Input: part model. Units: mm. Frame: model coordinates. Round coordinates to 2 decimals unless told otherwise and drop trailing zeros. Loops run counter-clockwise (first coordinate to the right, second up) from the corner with the lowest first, then second, coordinate; pieces in that order, holes last. Notation, with made-up numbers: (-10.5, 60) - (16.5, 60) arc R23 ccw to (16.5, 79) - close; hole circle Ø4 at (36.5, 39.5). An arc over 180 degrees is marked (long way). Write each question's results on one line, items separated by ' | '.
from build123d import *

# Parameters (mm, degrees)
SKETCH008_R      = 5
EXTRUDE002_DEPTH = 10


with BuildPart() as extrude002:
    # Sketch008 (on Face5 of Cut002) → Extrude002 (new body)
    with BuildSketch(Plane.XY.offset(1)):
        with Locations((35, 0)):
            Circle(SKETCH008_R)
        with Locations((0, 35)):
            Circle(SKETCH008_R)
        with Locations((-35, 0)):
            Circle(SKETCH008_R)
        with Locations((0, -35)):
            Circle(SKETCH008_R)
        with Locations((0, 55)):
            Circle(SKETCH008_R)
        with Locations((55, 0)):
            Circle(SKETCH008_R)
        with Locations((0, -55)):
            Circle(SKETCH008_R)
        with Locations((-55, 0)):
            Circle(SKETCH008_R)
        with Locations((-24.748737, 24.748737)):
            Circle(SKETCH008_R)
        with Locations((-24.748737, -24.748737)):
            Circle(SKETCH008_R)
        with Locations((24.748737, -24.748737)):
            Circle(SKETCH008_R)
        with Locations((24.748737, 24.748737)):
            Circle(SKETCH008_R)
        with Locations((-47.631397, 27.5)):
            Circle(SKETCH008_R)
        with Locations((-27.5, 47.631397)):
            Circle(SKETCH008_R)
        with Locations((27.5, 47.631397)):
            Circle(SKETCH008_R)
        with Locations((47.631397, 27.5)):
            Circle(SKETCH008_R)
        with Locations((47.631397, -27.5)):
            Circle(SKETCH008_R)
        with Locations((27.5, -47.631397)):
            Circle(SKETCH008_R)
        with Locations((-27.5, -47.631397)):
            Circle(SKETCH008_R)
        with Locations((-47.631397, -27.5)):
            Circle(SKETCH008_R)
    extrude(amount=-EXTRUDE002_DEPTH)


with BuildPart() as cone003:
    # Cone003 → Cone003 (revolve)
    with BuildSketch(Plane(origin=(0, 0, 1), x_dir=(1, 0, 0), z_dir=(0, -1, 0))):
        Polygon((0, 0), (69, 0), (70, 9), (0, 9), align=None)
    revolve(axis=Axis((0, 0, 1), (0, 0, 1)))


with BuildPart() as simple_bottom:
    # Cone002 → Cone002 (revolve)
    with BuildSketch(Plane.XZ):
        Polygon((0, 0), (70, 0), (71, 10), (0, 10), align=None)
    revolve(axis=Axis((0, 0, 0), (0, 0, 1)))

    # Cut002: cut Cone003
    add(cone003.part, mode=Mode.SUBTRACT)

    # Cut003: cut Extrude002
    add(extrude002.part, mode=Mode.SUBTRACT)


solid = simple_bottom.part
1. Section query A-A, the plane x = 0. Output: boundary loops of the cut face in (y, z), plus the area to 3 significant figures.
Answer:
outline: (-71, 10) - (-70, 0) - (-60, 0) - (-60, 1) - (-69, 1) - (-70, 10) - close; (-50, 0) - (-40, 0) - (-40, 1) - (-50, 1) - close; (-30, 0) - (30, 0) - (30, 1) - (-30, 1) - close; (40, 0) - (50, 0) - (50, 1) - (40, 1) - close; (60, 0) - (70, 0) - (71, 10) - (70, 10) - (69, 1) - (60, 1) - close | area: 119 mm^2
2. Line query: line 1 (X direction, y = -51, z = 0.5); line 2 (Y direction, x = 27.5, z = 0.6); line 3 (X direction, y = -49, z = 5). Output: solid intervals per line, ascending. Write a range as [from, to].
Answer:
line 1: [-48.02, -31.19], [-23.81, -3], [3, 23.81], [31.19, 48.02] | line 2: [-64.44, -52.63], [-42.63, -28.92], [-20.57, 20.57], [28.92, 42.63], [52.63, 64.44] | line 3: [-50.69, -49.21], [49.21, 50.69]
3. Contact query for flat-ended pins moving along their axis: pin 1 (2 mm diameter, centred on x = -43.5, z = 4.5, fed in from +Y); pin 2 (1.5 mm diameter, centred on x = -37, z = 6, fed in from +Y); pin 3 (5 mm diameter, centred on x = -4.5, y = 2.5, fed in from +Z). Output: stop coordinate, or through.
Answer:
pin 1: y = 56.2 | pin 2: y = 60.59 | pin 3: z = 1
4. Mould query, pull axis X, two halves, no side actions, for faces 1 (the conical face through (-69.995, 3.081, 0.626)), 2 (the cylindrical face through (-1.08, -39.88, 0.51)), 3 (the flat face through (1, 1, 0)). Classes: pulls with the +X half, pulls with the -X half, needs draft (parallel to the pull), parting line crosses it, or undercut.
Answer:
face 1: parting line crosses it | face 2: undercut | face 3: needs draft
5. Section query C-C, the plane z = 8.5. Output: boundary loops of the cut face in (x, y), plus the area to 3 significant figures.
Answer:
outline: circle Ø141.7 at (0, 0); hole circle Ø139.67 at (0, 0) | area: 449 mm^2
